Could you check a few things on this model? Use its own coordinates, in mm. Face numbers are marked on the shaded views. A direction names the side the tool comes from. Coordinates: 2 decimals unless noted, no trailing zeros. Loops run counter-clockwise (first coordinate to the right, second up) from the corner with the lowest first, then second, coordinate; pieces in that order, holes last. Notation, with made-up numbers: (85, 14.5) - (102, 14.5) arc R25 cw to (102, 44.5) - close; hole circle Ø11 at (48, -32). An arc over 180 degrees is marked (long way). One line per question, with ' | ' between items. Start each with the question number.
1. I want a section at B-B, the plane x = 24. Write out the boundary of the cut face in (y, z), then the cut area to 3 significant figures.
2. Please list where these lines run through material, in increasing order: L1, parallel to X at y = 3.75, z = 1.5; L2, parallel to X at y = 5.25, z = -19.5; L3, parallel to Y at x = 24, z = -2.25. Write a range as [from, to].
3. I want a section at D-D, the plane x = 31.5. Write out the boundary of the cut face in (y, z).
4. We'd pull the mould along Y, two halves only. Please class the marked faces 4, 5, 6 and 7: pulls with the +Y half, pulls with the -Y half, needs draft (parallel to the pull), parting line crosses it, or undercut.
5. I want a section at C-C, the plane y = -2. Write out the boundary of the cut face in (x, z).
6. I'm going to push flat-ended pins straight in: P1, Ø5, axis at x = 5, y = 3.5, coming from the -Z side; P2, Ø3, axis at x = 11.5, y = 4.5, coming from the +Z side; P3, Ø2, axis at x = 33.5, z = 4.5, coming from the +Y side. Where does each tip first touch, or does it pass through?
7. I want a section at A-A, the plane z = -14.5. Write out the boundary of the cut face in (x, y).
8. Which directions (+Z, -Z, +X, -X, +Y, -Y) give clear straight access to the entire face, cutting with the end or side of a thin tool? Please do the marked faces 1, 2 and 3.
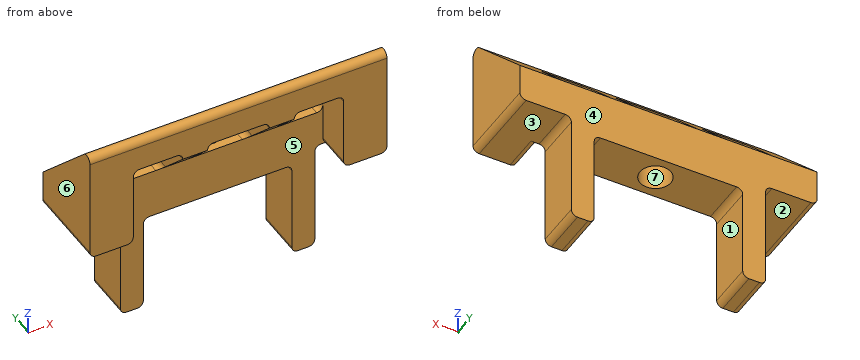
from build123d import *

# Parameters (mm, degrees)
BOSS_EXTRUDE2_DEPTH   = 7.5
BOSS_EXTRUDE3_DEPTH   = 48
BOSS_EXTRUDE4_DEPTH   = 7
CUT_EXTRUDE2_START    = -13.5
SKETCH4_W             = 8
SKETCH4_H             = 7
SKETCH4_W_2           = 10
CUT_EXTRUDE2_DEPTH    = 13.5
M6X1_0_TAPPED_HOLE4_D = 5
FILLET1_R             = 1


with BuildPart() as part:
    # Sketch1 → Boss-Extrude2 (new body)
    with BuildSketch(Plane(origin=(0, 0, 0), x_dir=(1, 0, 0), z_dir=(0, 1, 0))):
        Polygon((12, 24), (8.3, 24), (8.3, 6), (0, 6), (0, 0), (48, 0), (48, 6), (39.7, 6), (39.7, 24), (36, 24), (36, 8), (12, 8), align=None)
    extrude(amount=BOSS_EXTRUDE2_DEPTH)

    # Sketch3 → Boss-Extrude3 (add)
    with BuildSketch(Plane(origin=(48, 0, 0), x_dir=(0, 0, -1), z_dir=(1, 0, 0))):
        Polygon((0, 0), (-6, -6), (-13.5, -6), (0, 7.5), align=None)
    extrude(amount=-BOSS_EXTRUDE3_DEPTH)

    # Sketch16 → Boss-Extrude4 (add)
    with BuildSketch(Plane(origin=(48, 0, 0), x_dir=(0, 0, -1), z_dir=(1, 0, 0))):
        Polygon((-6, -6), (6, -6), (6, 0), (0, 0), align=None)
    boss_extrude4 = extrude(amount=-BOSS_EXTRUDE4_DEPTH)

    # Sketch4 → Cut-Extrude2 (cut)
    with BuildSketch(Plane.XZ.offset(6).offset(CUT_EXTRUDE2_START)):
        with Locations((11, 3.5)):
            Rectangle(SKETCH4_W, SKETCH4_H)
        with Locations((37, 3.5)):
            Rectangle(SKETCH4_W, SKETCH4_H)
        with Locations((24, 3.5)):
            Rectangle(SKETCH4_W_2, SKETCH4_H)
    extrude(amount=CUT_EXTRUDE2_DEPTH, mode=Mode.SUBTRACT)

    # M6x1.0 Tapped Hole4 (through all)
    with Locations(Plane(origin=(0, 0, -8), x_dir=(-1, 0, 0), z_dir=(0, 0, -1))):
        with Locations((-24, 3.75)):
            Hole(M6X1_0_TAPPED_HOLE4_D / 2)

    # Mirror1: Boss-Extrude4 across plane
    add(boss_extrude4.mirror(Plane.ZY.offset(-24)))

    # Fillet1
    fillet1_edges = [part.edges().sort_by_distance(p)[0] for p in [
        (29, 3.75, 0),
        (29, -2.75, 7),
        (19, -2.75, 7),
        (19, 3.75, 0),
        (7, -3, -6),
        (39.7, 3.75, -24),
        (39.7, 3.75, -6),
        (48, 0.75, -6),
        (0, 0.75, -6),
        (8.3, 3.75, -6),
        (8.3, 3.75, -24),
        (12, 3.75, -24),
        (12, 3.75, -8),
        (36, 3.75, -8),
        (36, 3.75, -24),
        (24, -6, 13.5),
        (41, -3, -6),
        (15, 3.75, 0),
        (15, -2.75, 7),
        (7, -2.75, 7),
        (7, 3.75, 0),
        (33, -2.75, 7),
        (33, 3.75, 0),
        (41, 3.75, 0),
        (41, -2.75, 7),
    ]]
    fillet(fillet1_edges, radius=FILLET1_R)


solid = part.part
Results are:
1) outline: (-6, 7) - (0.5, 7) - (-4.29, 11.79) arc R1 ccw to (-6, 11.09) - close; (0, -8) - (1.25, -8) - (1.25, 0) - (0, 0) - close; (6.25, -8) - (7.5, -8) - (7.5, 0) - (6.25, 0) - close | area: 39.9 mm2
2) L1: x = [0, 7], [15, 19], [29, 33], [41, 48] | L2: x = [8.3, 12], [36, 39.7] | L3: y = [0, 1.25], [6.25, 7.5]
3) outline: (-6, 6) - (0, 0) - (0, -8) - (7.5, -8) - (7.5, 0) - (-4.29, 11.79) arc R1 ccw to (-6, 11.09) - close
4) face 4: pulls with the +Y half | face 5: pulls with the -Y half | face 6: needs draft | face 7: undercut
5) outline: (0, -5) arc R1 ccw to (1, -6) - (6, -6) arc R1 ccw to (7, -5) - (7, 6) arc R1 cw to (8, 7) - (14, 7) arc R1 cw to (15, 6) - (15, 2) - (19, 2) - (19, 6) arc R1 cw to (20, 7) - (28, 7) arc R1 cw to (29, 6) - (29, 2) - (33, 2) - (33, 6) arc R1 cw to (34, 7) - (40, 7) arc R1 cw to (41, 6) - (41, -5) arc R1 ccw to (42, -6) - (47, -6) arc R1 ccw to (48, -5) - (48, 9.5) - (0, 9.5) - close
6) P1: stops at z = -6.02 | P2: stops at z = 0 | P3: stops at y = 3.87
7) outline: (8.3, 0) - (12, 0) - (12, 7.5) - (8.3, 7.5) - close; (36, 0) - (39.7, 0) - (39.7, 7.5) - (36, 7.5) - close
8) face 1: -Z, +Y, -Y | face 2: -Z, -X, +Y, -Y | face 3: -Z, +X, +Y, -Y
